Build history of the part. All positions in model axes, mm. Coordinates: 2 decimals unless noted, no trailing zeros. Loops run counter-clockwise (first coordinate to the right, second up) from the corner with the lowest first, then second, coordinate; pieces in that order, holes last. Notation, with made-up numbers: (-5, -20.75) - (49, -20.75) arc R21 ccw to (49, -11.75) - close; hole circle Ø4 at (68, 40.5). An arc over 180 degrees is marked (long way). One line per item, written item: value.
```python
from build123d import *

# Parameters (mm, degrees)
SKICA1_W                 = 16
SKICA1_H                 = 16
SKICA1_R                 = 3
P_IDAT_VYSUNUT_M1_DEPTH  = 12
SKICA2_R                 = 2.5
ODEBRAT_VYSUNUT_M1_DEPTH = 22


with BuildPart() as part:
    # Skica1 → Přidat vysunutím1 (new body)
    with BuildSketch(Plane(origin=(0, 0, 0), x_dir=(1, 0, 0), z_dir=(0, 1, 0))):
        Rectangle(SKICA1_W, SKICA1_H)
        with Locations(Location((-3, 0, 0), (0, 0, 270))):
            Circle(SKICA1_R, mode=Mode.SUBTRACT)
    extrude(amount=P_IDAT_VYSUNUT_M1_DEPTH)

    # Skica2 → Odebrat vysunutím1 (cut)
    with BuildSketch(Plane.XY.offset(8)):
        with Locations((4, 6)):
            Circle(SKICA2_R)
    extrude(amount=-ODEBRAT_VYSUNUT_M1_DEPTH, mode=Mode.SUBTRACT)


solid = part.part
```
Item 1: Cut at C-C, the plane y = 5.75. Write the cut outline in (x, z), then the cut area to 3 significant figures.
Check result:
outline: (-8, -8) - (1.51, -8) - (1.51, 8) - (-8, 8) - close; (6.49, -8) - (8, -8) - (8, 8) - (6.49, 8) - close; hole circle Ø6 at (-3, 0)
area: 148 mm^2
Item 2: Pull direction Y, two halves, no side cores. Call faces 1 (the face through (6.385, 6.751, 0.112)), 2 (the face through (2, 0, 0)), 3 (the face through (-8, 6, 0)): released by +Y, released by -Y, zero draft, split by the parting line, or undercut.
Check result:
face 1: undercut
face 2: released by -Y
face 3: zero draft
Item 3: Cut at B-B, the plane x = 2. Write the cut outline in (y, z).
Check result:
outline: (0, -8) - (4.5, -8) - (4.5, 8) - (0, 8) - close; (7.5, -8) - (12, -8) - (12, 8) - (7.5, 8) - close
Item 4: Probe probe 1 along Y at (x, z) = (4, -5.5); probe 2 along X at (y, z) = (7.75, 0); probe 3 along Y at (x, z) = (2.25, 4.25). List the from-to ranges inside material, lowest first. Write a range as from..to.
Check result:
probe 1: y = 0..3.5, 8.5..12
probe 2: x = -8..-6, 0..2.21, 5.79..8
probe 3: y = 0..4.21, 7.79..12
Item 5: Cut at A-A, the plane z = 0. Write the cut outline in (x, y), then the cut area to 3 significant figures.
Check result:
outline: (-8, 0) - (-6, 0) - (-6, 12) - (-8, 12) - close; (0, 0) - (8, 0) - (8, 12) - (0, 12) - close; hole circle Ø5 at (4, 6)
area: 100 mm^2
Item 6: Cut at D-D, the plane y = 1.5. Write the cut outline in (x, z), then the cut area to 3 significant figures.
Check result:
outline: (-8, -8) - (8, -8) - (8, 8) - (-8, 8) - close; hole circle Ø6 at (-3, 0)
area: 228 mm^2
